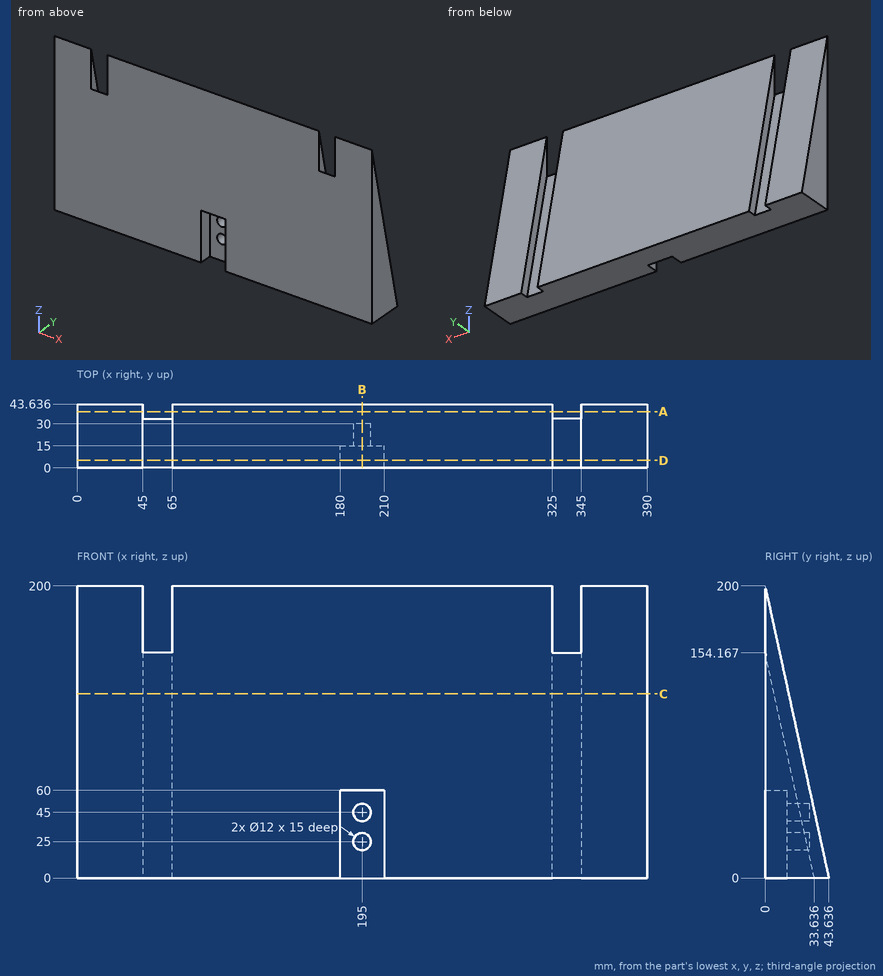
Study the drawing (mm; zero at the part's minimum x, y, z) and answer. Round coordinates to 2 decimals unless told otherwise and drop trailing zeros. Write each loop counter-clockwise with the first axis right and the second up, starting at its lowest first coordinate (ties: lowest second). Pieces come first, ordered by that corner, then holes.
Q1. Find section C-C on z = 126. Determine the outline of the cut face in (x, y) (1 decimal).
Values:
outline: (0, 0) - (390, 0) - (390, 16.1) - (345, 16.1) - (345, 6.1) - (325, 6.1) - (325, 16.1) - (65, 16.1) - (65, 6.1) - (45, 6.1) - (45, 16.1) - (0, 16.1) - close
Q2. Straight lines are drawn through the part: line 1 (X direction, y = 7.5, z = 145.5); line 2 (X direction, y = 4.5, z = 21); line 3 (X direction, y = 16.5, z = 39.5) (1 decimal). For each, find the intervals that lie inside material, in ascending order.
Values:
line 1: x = 0 to 45, 65 to 325, 345 to 390
line 2: x = 0 to 180, 210 to 390
line 3: x = 0 to 192.6, 197.4 to 390
Q3. Find section B-B on x = 195. Determine the outline of the cut face in (y, z), and give its area (3 significant figures).
Values:
outline: (0, 60) - (15, 60) - (15, 51) - (30, 51) - (30, 39) - (15, 39) - (15, 31) - (30, 31) - (30, 19) - (15, 19) - (15, 0) - (43.64, 0) - (0, 200) - close
area: 3,100 mm2
Q4. Find section A-A on y = 38.5. Determine the outline of the cut face in (x, z), and give its area (3 significant figures).
Values:
outline: (0, 0) - (45, 0) - (45, 23.54) - (0, 23.54) - close; (65, 0) - (325, 0) - (325, 23.54) - (65, 23.54) - close; (345, 0) - (390, 0) - (390, 23.54) - (345, 23.54) - close
area: 8,240 mm2
Q5. Flat-ended cylindrical pins translate along their axes: P1, Ø3.5, axis at x = 194, z = 44, coming from the -Y side; P2, Ø11, axis at x = 195, z = 25, coming from the +Y side; P3, Ø8, axis at x = 343, z = 76, coming from the +Y side. Find the tip coordinate at first contact, or state that the pin passes through.
Values:
P1: stops at y = 30
P2: stops at y = 39.38
P3: stops at y = 27.81
Q6. Find section D-D on y = 5. Determine the outline of the cut face in (x, z).
Values:
outline: (0, 0) - (180, 0) - (180, 60) - (210, 60) - (210, 0) - (390, 0) - (390, 177.08) - (345, 177.08) - (345, 131.25) - (325, 131.25) - (325, 177.08) - (65, 177.08) - (65, 131.25) - (45, 131.25) - (45, 177.08) - (0, 177.08) - close
